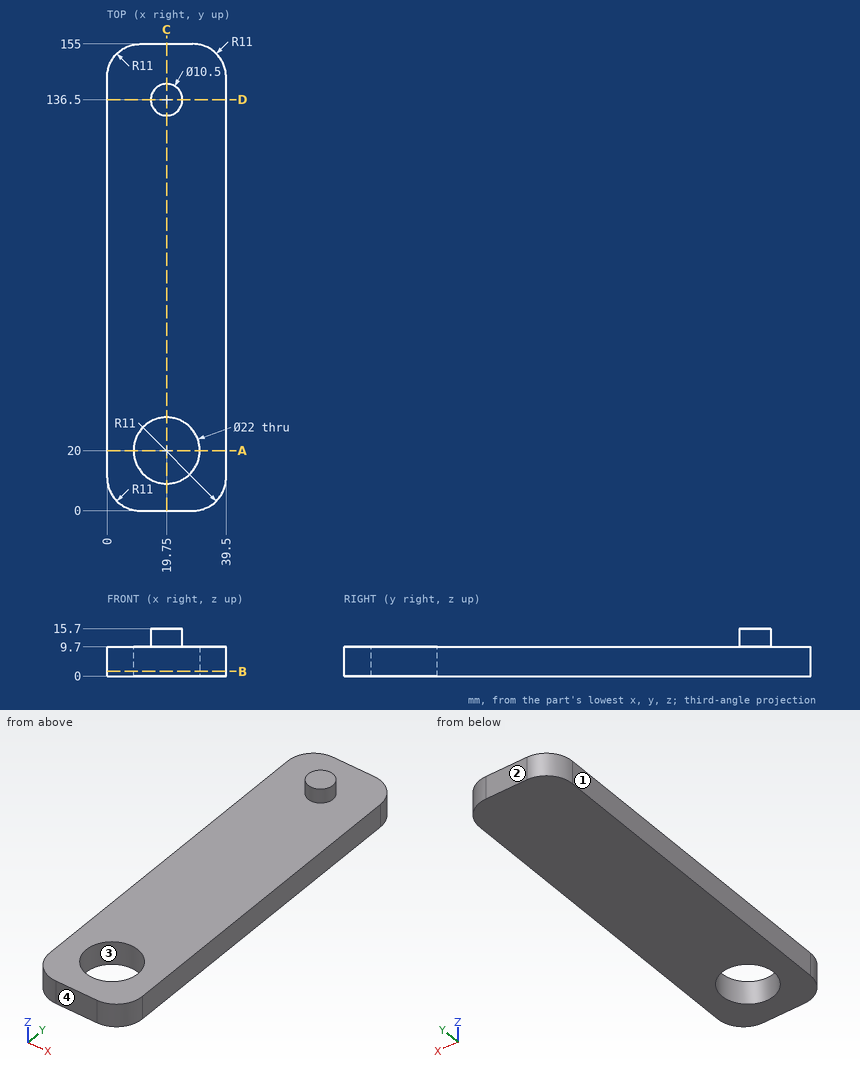
Part print with two shaded views. Sizes in mm from the minimum x, y, z corner. Coordinates: 2 decimals unless noted, no trailing zeros. Order: outer loops, then holes, each group sorted by start corner. A loop starts at its lowest first (then second) coordinate and runs counter-clockwise, first axis right, second up. Notation, with made-up numbers: M 65,82 L 70,82 A16 cw 70,99 Z; hole C -20,15.25 d4. An arc over 180 degrees is marked long. One line per question, with ' | ' between items. Start each with the question number.
1. Cut at D-D (y = 136.5). Write the cut outline in (x, z), plus the area to 3 significant figures.
2. Cut at B-B (z = 1.5). Write the cut outline in (x, y).
3. Cut at C-C (x = 19.75). Write the cut outline in (y, z).
4. Wall check: line 1 along Y through (x, z) = (19.75, 6.5); line 2 along Z through (x, y) = (23.5, 126); line 3 along Y through (x, z) = (21.5, 8). Give the ranges that are in metal, low to high. Write a range as [from, to].
5. Cut at A-A (y = 20). Write the cut outline in (x, z).
6. Flat gauge pin, fed straight in: P1, Ø1.5, axis at x = 32.5, z = 4.5, coming from the -Y side. Where does the tip first touch, or does it go through?
7. Mould opens along Y. For the marked faces 1, 2, 3 and 4 say: +Y half, -Y half, draft (parallel to the pull), parting line (faces both ways), or undercut.
The answers:
1) outline: M 0,0 L 39.5,0 L 39.5,9.7 L 25,9.7 L 25,15.7 L 14.5,15.7 L 14.5,9.7 L 0,9.7 Z | area: 446 mm2
2) outline: M 0,11 A11 ccw 11,0 L 28.5,0 A11 ccw 39.5,11 L 39.5,144 A11 ccw 28.5,155 L 11,155 A11 ccw 0,144 Z; hole C 19.75,20 d22
3) outline: M 0,0 L 9,0 L 9,9.7 L 0,9.7 Z; M 31,0 L 155,0 L 155,9.7 L 141.75,9.7 L 141.75,15.7 L 131.25,15.7 L 131.25,9.7 L 31,9.7 Z
4) line 1: y = [0, 9], [31, 155] | line 2: z = [0, 9.7] | line 3: y = [0, 9.14], [30.86, 155]
5) outline: M 0,0 L 8.75,0 L 8.75,9.7 L 0,9.7 Z; M 30.75,0 L 39.5,0 L 39.5,9.7 L 30.75,9.7 Z
6) P1: stops at y = 0.49
7) face 1: draft | face 2: +Y half | face 3: undercut | face 4: -Y half
